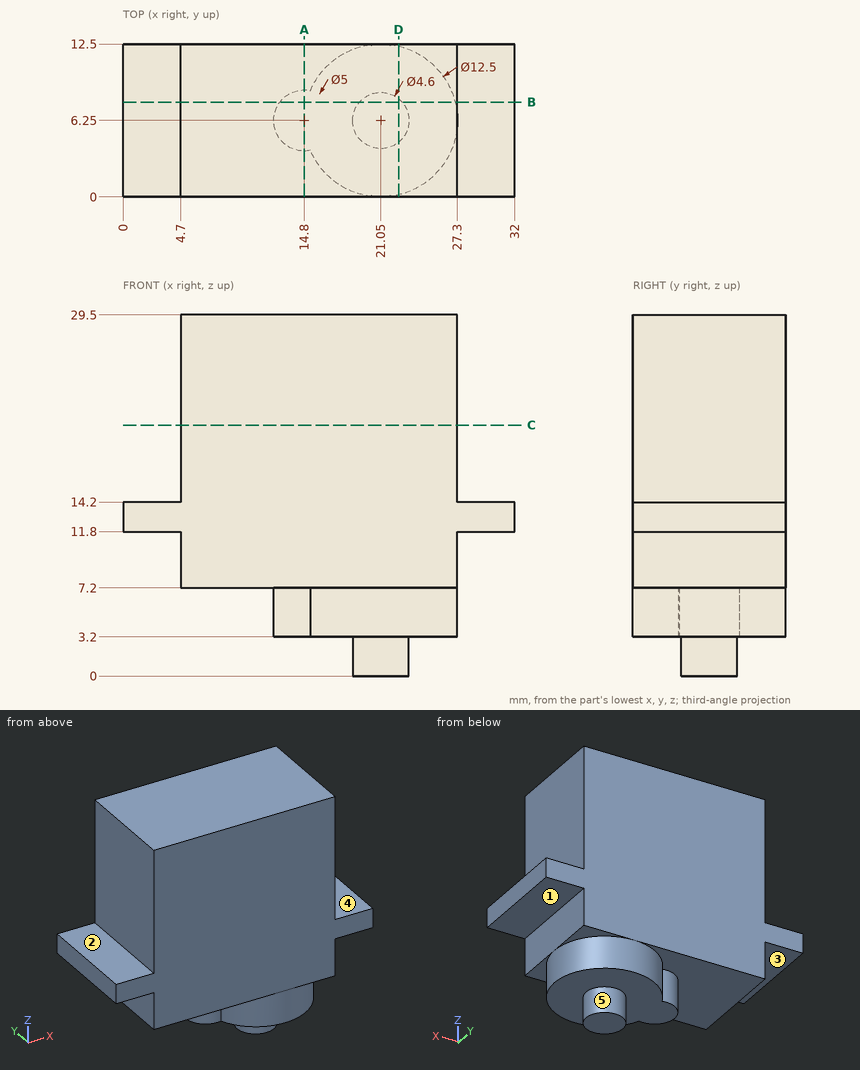
Here's the drawing with two shaded views (mm, measured from the low corner). I have some questions. A direction names the side the tool comes from. Round coordinates to 2 decimals unless told otherwise and drop trailing zeros. Loops run counter-clockwise (first coordinate to the right, second up) from the corner with the lowest first, then second, coordinate; pieces in that order, holes last. Notation, with made-up numbers: (69, 71.25) - (101, 71.25) arc R20 cw to (101, 103.25) - close; hole circle Ø7 at (41, -6). An arc over 180 degrees is marked (long way). Use CSV: the item, a comma, the result in double quotes.
Item 1: For the marked faces 1, 2, 3, 4 and 5, which set-ups out of +Z, -Z, +X, -X, +Y, -Y let a thin tool reach every point of the face, with its end or its side?
Here are the results:
face 1,"-Z, +X, +Y, -Y"
face 2,"+Z, -X, +Y, -Y"
face 3,"-Z, -X, +Y, -Y"
face 4,"+Z, +X, +Y, -Y"
face 5,"-Z"
Item 2: If we section it at D-D on x = 22.5: List the corners of the cut face in (y, z) for me, then the cut area to 3 significant figures.
Here are the results:
outline,"(0, 7.2) - (0.17, 7.2) - (0.17, 3.2) - (4.46, 3.2) - (4.46, 0) - (8.04, 0) - (8.04, 3.2) - (12.33, 3.2) - (12.33, 7.2) - (12.5, 7.2) - (12.5, 29.5) - (0, 29.5) - close"
area,"339 mm²"
Item 3: If we section it at C-C on z = 20.5: List the corners of the cut face in (x, y) for me.
Here are the results:
outline,"(4.7, 0) - (27.3, 0) - (27.3, 12.5) - (4.7, 12.5) - close"
Item 4: Will these pins go through, and if not, where does the flat tip stop? pin 1 (1.9 mm diameter, centred on x = 25.5, y = 3.5, fed in from -Z); pin 2 (1 mm diameter, centred on y = 10.5, z = 23.5, fed in from -X); pin 3 (3 mm diameter, centred on y = 8, z = 8.5, fed in from +X).
Here are the results:
pin 1,"stops at z = 3.2"
pin 2,"stops at x = 4.7"
pin 3,"stops at x = 27.3"
Item 5: I need wall thicknesses on L1, parallel to Z at x = 23.5, y = 4.5; L2, parallel to Z at x = 27, y = 0.75; L3, parallel to X at y = 6.5, z = 11.5. Which ranges of each line are inside material? Lowest first, please. Write a range as [from, to].
Here are the results:
L1,"z = [3.2, 29.5]"
L2,"z = [7.2, 29.5]"
L3,"x = [4.7, 27.3]"
Item 6: If we section it at B-B on y = 7.75: List the corners of the cut face in (x, z) for me.
Here are the results:
outline,"(0, 11.8) - (4.7, 11.8) - (4.7, 7.2) - (12.8, 7.2) - (12.8, 3.2) - (19.31, 3.2) - (19.31, 0) - (22.79, 0) - (22.79, 3.2) - (27.12, 3.2) - (27.12, 7.2) - (27.3, 7.2) - (27.3, 11.8) - (32, 11.8) - (32, 14.2) - (27.3, 14.2) - (27.3, 29.5) - (4.7, 29.5) - (4.7, 14.2) - (0, 14.2) - close"
Item 7: If we section it at A-A on x = 14.8: List the corners of the cut face in (y, z) for me, then the cut area to 3 significant figures.
Here are the results:
outline,"(0, 7.2) - (3.75, 7.2) - (3.75, 3.2) - (8.75, 3.2) - (8.75, 7.2) - (12.5, 7.2) - (12.5, 29.5) - (0, 29.5) - close"
area,"299 mm²"
